The listing builds one solid part. Answer for the finished solid, in the listing's coordinates (mm). A direction names the side the tool comes from. Give positions to 0.01 mm unless a question says otherwise; leave off trailing zeros. Write each loop counter-clockwise with the first axis right and the second up, starting at its lowest first coordinate (ties: lowest second). Pieces come first, ordered by that corner, then holes. Notation, with made-up numbers: (67, -17) -> (72, -17) arc R29 cw to (72, 12) -> close; hole circle Ø6 at (-24, 84). An arc over 180 degrees is marked (long way). Write each question's results on one line, items separated by ' | '. Start each with the question number.
from build123d import *

# Parameters (mm, degrees)
F0_R      = 73.096751
F1_DEPTH  = 25.4
F2_R      = 6.35
F3_DEPTH  = 25.4
F4_R      = 14.2875
F4_R_2    = 6.35
F5_DEPTH  = 9.525
F6_R      = 9.525
F7_DEPTH  = 9.525
F8_R      = 22.225
F9_DEPTH  = 25.4
F10_R     = 12.7
F11_DEPTH = 12.7


with BuildPart() as f1:
    # F0 (on Front) → F1 (new body)
    with BuildSketch(Plane.XZ):
        Circle(F0_R)
    extrude(amount=F1_DEPTH)

    # F2 (on face) → F3 (cut)
    with BuildSketch(Plane(origin=(0, 0, 0), x_dir=(-1, 0, 0), z_dir=(0, 1, 0))):
        with Locations((0, 50.8)):
            Circle(F2_R)
    extrude(amount=-F3_DEPTH, mode=Mode.SUBTRACT)

    # F4 (on face) → F5 (join)
    with BuildSketch(Plane(origin=(0, 0, 0), x_dir=(-1, 0, 0), z_dir=(0, 1, 0))):
        with Locations((0, 50.8)):
            Circle(F4_R)
        with Locations((0, 50.8)):
            Circle(F4_R_2, mode=Mode.SUBTRACT)
    extrude(amount=F5_DEPTH)

    # F6 (on face) → F7 (cut)
    with BuildSketch(Plane(origin=(0, 9.525, 0), x_dir=(-1, 0, 0), z_dir=(0, 1, 0))):
        with Locations((0, 50.8)):
            Circle(F6_R)
    extrude(amount=-F7_DEPTH, mode=Mode.SUBTRACT)

    # F8 (on face) → F9 (cut)
    with BuildSketch(Plane(origin=(0, 0, 0), x_dir=(-1, 0, 0), z_dir=(0, 1, 0))):
        Circle(F8_R)
    extrude(amount=-F9_DEPTH, mode=Mode.SUBTRACT)

    # F10 (on face) → F11 (cut)
    with BuildSketch(Plane.XZ.offset(25.4)):
        with Locations((0, 50.8)):
            Circle(F10_R)
    extrude(amount=-F11_DEPTH, mode=Mode.SUBTRACT)


solid = f1.part
1. Section A-A (x = 0) is taken. Give the number of separate pieces and of enclosed holes in the cut face, then the cut area to 3 significant figures.
2. Each of these flat-tipped pins is pushed along its axis until it touches: pin 1 Ø4 at (y, z) = (-6.5, 16) entering from +X; pin 2 Ø17 at (x, z) = (0, 50.8) entering from -Y; pin 3 Ø16.5 at (x, z) = (0, 50.8) entering from +Y. Where does it stop, or does it pass through?
3. A tool of negligible diameter and unlimited length cuts with its end or side. For faces 5 (the flat face through (-6, -12.7, 48)), 6 (the cylindrical face through (0.8, -6.4, 57.1)), 7 (the flat face through (-6.2, 0, 48.8)), from which of +Z, -Z, +X, -X, +Y, -Y can it reach the whole face along a straight path? Write none if from no direction.
4. Section B-B (z = 0) is taken. Write down the section's boundary in (x, y) (3 decimals).
5. Consider probe 1 along Z at (x, y) = (0, -20) (3 decimals); probe 2 along Z at (x, y) = (0, -11) (3 decimals); probe 3 along X at (y, z) = (5, 50). Determine where each line is inside the solid, lowest interval first. Write a range as [from, to].
6. The mould has two halves that part along Z. Classify faces 1 (the cylindrical face through (5.86, -19.139, 39.533)), 2 (the flat face through (-3, 9.525, 41)), 3 (the cylindrical face through (1.86, 4.696, 64.966)), 4 (the cylindrical face through (1.24, 4.829, 60.244)): pulls with the +Z half, pulls with the -Z half, needs draft (parallel to the pull), parting line crosses it, or undercut.
Results:
1) separate pieces: 3 | enclosed holes: 0 | area: 2,190 mm²
2) pin 1: stops at x = 71.74 | pin 2: stops at y = -12.7 | pin 3: stops at y = 0
3) face 5: -Y | face 6: +Y, -Y | face 7: +Y
4) outline: (-73.097, -25.4) -> (-22.225, -25.4) -> (-22.225, 0) -> (-73.097, 0) -> close; (22.225, -25.4) -> (73.097, -25.4) -> (73.097, 0) -> (22.225, 0) -> close
5) probe 1: z = [-73.097, -22.225], [22.225, 38.1], [63.5, 73.097] | probe 2: z = [-73.097, -22.225], [22.225, 44.45], [57.15, 73.097] | probe 3: x = [-14.27, -9.49], [9.49, 14.27]
6) face 1: undercut | face 2: needs draft | face 3: parting line crosses it | face 4: undercut
